from build123d import *

# Parameters (mm, degrees)
BOSS_EXTRUDE1_START = -170
BOSS_EXTRUDE1_DEPTH = 5
BOSS_EXTRUDE2_START = -165
SKETCH3_4_W         = 5
SKETCH3_4_H         = 5
BOSS_EXTRUDE2_DEPTH = 30
BOSS_EXTRUDE3_START = -135
SKETCH3_5_W         = 50
SKETCH3_5_H         = 220
BOSS_EXTRUDE3_DEPTH = 5
BOSS_EXTRUDE4_START = -130
SKETCH3_6_W         = 5
SKETCH3_6_H         = 5
SKETCH3_6_W_2       = 50
BOSS_EXTRUDE4_DEPTH = 130
SKETCH6_R           = 8.5
CUT_EXTRUDE1_DEPTH  = 347.121365998


with BuildPart() as part:
    # Sketch3 → Boss-Extrude1 (new body)
    with BuildSketch(Plane(origin=(0, 0, 0), x_dir=(0, 0, -1), z_dir=(1, 0, 0)).offset(BOSS_EXTRUDE1_START)):
        with BuildLine():
            Line((-30, 0), (-30, 300))
            Line((-30, 300), (30, 300))
            Line((30, 300), (30, 0))
            ThreePointArc((30, 0), (0, -30), (-30, 0))
        make_face()
    extrude(amount=BOSS_EXTRUDE1_DEPTH)

    # Sketch3<4> → Boss-Extrude2 (add)
    with BuildSketch(Plane(origin=(0, 0, 0), x_dir=(0, 0, -1), z_dir=(1, 0, 0)).offset(BOSS_EXTRUDE2_START)):
        Polygon((-30, 75), (-25, 75), (-25, 295), (25, 295), (25, 75), (30, 75), (30, 300), (-30, 300), align=None)
        with Locations((-27.5, 72.5)):
            Rectangle(SKETCH3_4_W, SKETCH3_4_H)
        with BuildLine():
            Line((0, -30), (0, -25))
            ThreePointArc((0, -25), (-17.67766953, -17.67766953), (-25, 0))
            Line((-25, 0), (-25, 70))
            Line((-25, 70), (-30, 70))
            Line((-30, 70), (-30, 0))
            ThreePointArc((-30, 0), (-21.213203436, -21.213203436), (0, -30))
        make_face()
        with Locations((27.5, 72.5)):
            Rectangle(SKETCH3_4_W, SKETCH3_4_H)
        with BuildLine():
            ThreePointArc((25, 0), (17.67766953, -17.67766953), (0, -25))
            Line((0, -25), (0, -30))
            ThreePointArc((0, -30), (21.213203436, -21.213203436), (30, 0))
            Line((30, 0), (30, 70))
            Line((30, 70), (25, 70))
            Line((25, 70), (25, 0))
        make_face()
    extrude(amount=BOSS_EXTRUDE2_DEPTH)

    # Sketch3<5> → Boss-Extrude3 (add)
    with BuildSketch(Plane(origin=(0, 0, 0), x_dir=(0, 0, -1), z_dir=(1, 0, 0)).offset(BOSS_EXTRUDE3_START)):
        with BuildLine():
            ThreePointArc((-30, 0), (0, -30), (30, 0))
            Line((30, 0), (30, 300))
            Line((30, 300), (-30, 300))
            Line((-30, 300), (-30, 0))
        make_face()
        with Locations((0, 185)):
            Rectangle(SKETCH3_5_W, SKETCH3_5_H, mode=Mode.SUBTRACT)
    extrude(amount=BOSS_EXTRUDE3_DEPTH)

    # Sketch3<6> → Boss-Extrude4 (add)
    with BuildSketch(Plane(origin=(0, 0, 0), x_dir=(0, 0, -1), z_dir=(1, 0, 0)).offset(BOSS_EXTRUDE4_START)):
        Polygon((-30, 300), (-30, 75), (-25, 75), (-25, 295), (25, 295), (25, 75), (30, 75), (30, 300), align=None)
        with Locations((-27.5, 72.5)):
            Rectangle(SKETCH3_6_W, SKETCH3_6_H)
        with Locations((0, 72.5)):
            Rectangle(SKETCH3_6_W_2, SKETCH3_6_H)
        with Locations((27.5, 72.5)):
            Rectangle(SKETCH3_6_W, SKETCH3_6_H)
    extrude(amount=BOSS_EXTRUDE4_DEPTH)

    # Sketch6 → Cut-Extrude1 (cut, through all)
    with BuildSketch(Plane(origin=(0, 0, 0), x_dir=(0, 0, -1), z_dir=(1, 0, 0))):
        Circle(SKETCH6_R)
    extrude(amount=-CUT_EXTRUDE1_DEPTH, mode=Mode.SUBTRACT)

    # Mirror5: part across plane


with BuildPart() as part_1:
    add(part.part)
    add(part.part.mirror(Plane(origin=(0, 0, 0), x_dir=(0, 0, 1), z_dir=(1, 0, 0))))


solid = part_1.part
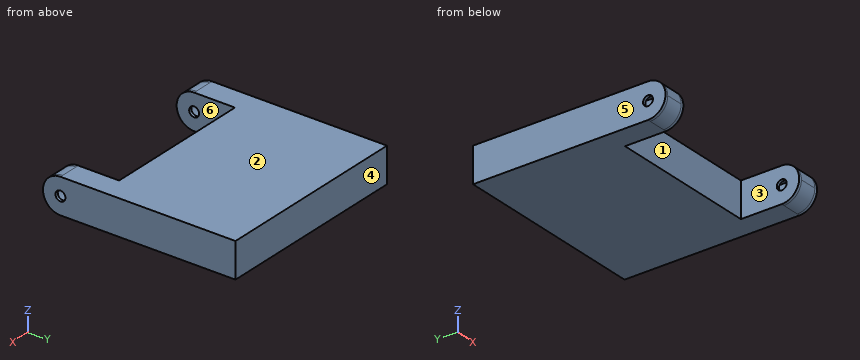
Build history of the part. All positions in model axes, mm. Face numbers are marked on the shaded views. A direction names the side the tool comes from. Coordinates: 2 decimals unless noted, no trailing zeros. Order: outer loops, then holes, each group sorted by start corner. A loop starts at its lowest first (then second) coordinate and runs counter-clockwise, first axis right, second up. Notation, with made-up numbers: (-16.5, 2) - (2.5, 2) arc R25 cw to (2.5, 28) - close; hole circle Ø10 at (74, -13.75). An arc over 180 degrees is marked (long way). Put each result on its own line as item: value.
1. Pull direction X, two halves, no side cores. Call the marked faces 3, 4, 5 and 6: pulls with the +X half, pulls with the -X half, needs draft (parallel to the pull), parting line crosses it, or undercut.
Answer sheet:
face 3: undercut
face 4: needs draft
face 5: pulls with the -X half
face 6: undercut
2. Saw through at A-A (y = 43). Write the cut outline in (x, z).
Answer sheet:
outline: (-170, -30) - (-130, -30) - (-130, 30) - (-170, 30) - close; (130, -30) - (170, -30) - (170, 30) - (130, 30) - close; hole (-165, -25) - (-135, -25) - (-135, 25) - (-165, 25) - close; hole (135, -25) - (165, -25) - (165, 25) - (135, 25) - close
3. Saw through at B-B (x = -56). Write the cut outline in (y, z).
Answer sheet:
outline: (70, -30) - (300, -30) - (300, 30) - (70, 30) - close; hole (75, -25) - (295, -25) - (295, 25) - (75, 25) - close
4. Saw through at D-D (z = -16.5). Write the cut outline in (x, y).
Answer sheet:
outline: (-170, -25.05) - (-130, -25.05) - (-130, 70) - (130, 70) - (130, -25.05) - (170, -25.05) - (170, 300) - (-170, 300) - close; hole (-165, -18.78) - (-135, -18.78) - (-135, 75) - (135, 75) - (135, -18.78) - (165, -18.78) - (165, 295) - (-165, 295) - close
5. Saw through at C-C (y = 235.5). Write the cut outline in (x, z).
Answer sheet:
outline: (-170, -30) - (170, -30) - (170, 30) - (-170, 30) - close; hole (-165, -25) - (165, -25) - (165, 25) - (-165, 25) - close
6. Tool access for the marked faces 1 and 2: list every direction of +Z, -Z, +X, -X, +Y, -Y with a clear straight run to the whole face (end or side of a thin tool).
Answer sheet:
face 1: +Z, -Z, -Y
face 2: +Z, +X, -X, +Y, -Y
7. Probe line 1 along Y through (x, z) = (-132, 0); line 2 along X through (y, z) = (-16, 6.5); line 3 along Y through (x, z) = (-133, -1). List the from-to ranges inside material, lowest first. Write a range as [from, to].
Answer sheet:
line 1: y = [-30, -8.5], [8.5, 75], [295, 300]
line 2: x = [-170, -165], [-135, -130], [130, 135], [165, 170]
line 3: y = [-29.98, -8.44], [8.44, 75], [295, 300]
8. Drop a flat-ended pin along its axis: P1, Ø15, axis at x = 23.5, z = 6, coming from the -Y side. Give the stop position or say it passes through.
Answer sheet:
P1: stops at y = 70
